The drawing under review shows one solid part. Ordinate dimensions are in mm from its lowest x, y, z. A direction names the side the tool comes from. Give positions to 0.01 mm unless a question says otherwise; leave off trailing zeros. Write each loop counter-clockwise with the first axis right and the second up, starting at its lowest first coordinate (ties: lowest second). Pieces come first, ordered by that corner, then holes. Notation, with made-up numbers: M 64.5,46.25 L 114.5,46.25 A23 ccw 114.5,60.25 Z; hole C -40,58 d2. An arc over 180 degrees is marked long. One line per item, written item: value. Start each with the question number.
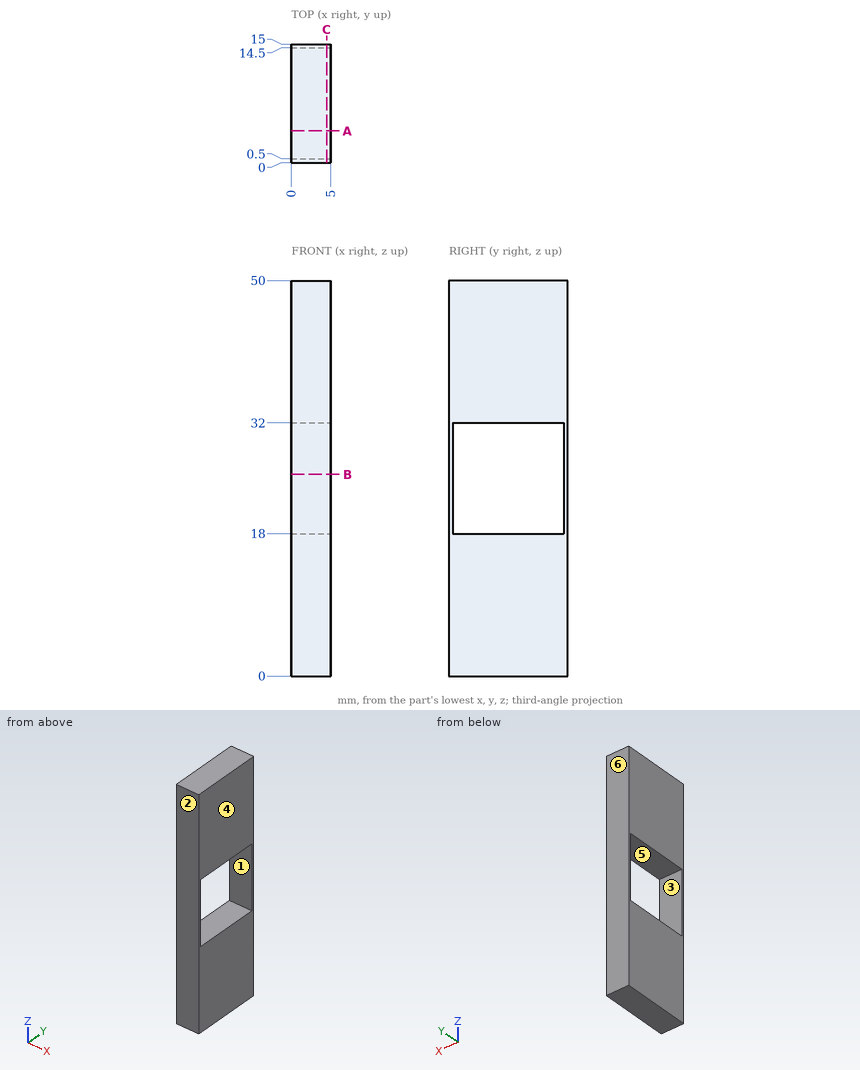
Q1. Take a section at B-B, the plane z = 25.5. Give the boundary of the cut face in (x, y).
Q2. For P1, Ø2, axis at y = 12, z = 39.5, coming from the -X side; P2, Ø1.5, axis at y = 5.5, z = 19, coming from the +X side, all flat-tipped, find the tip position at first contact; note any pin that passes through.
Q3. Take a section at C-C, the plane x = 4.45. Give the boundary of the cut face in (y, z), then the cut area to 3 significant figures.
Q4. Wall thickness on line 1 (Z direction, x = 4.35, y = 8.25); line 2 (Y direction, x = 4.1, z = 27): over which ranges is each line inside the solid? List them lowest first. Write a range as from..to.
Q5. The part is to be moulded in two halves that separate along Y. For the marked faces 1, 2, 3 and 4, say which applies: pulls with the +Y half, pulls with the -Y half, needs draft (parallel to the pull), parting line crosses it, or undercut.
Q6. Machinability: for the marked faces 5 and 6, which of the approach directions +Z, -Z, +X, -X, +Y, -Y give a long, thin tool a straight path to every point of the face, cutting with its end or side? Answer none if there is none.
Q7. Take a section at A-A, the plane y = 4. Give the boundary of the cut face in (x, z), then the cut area to 3 significant figures.
Results list:
1. outline: M 0,0 L 5,0 L 5,0.5 L 0,0.5 Z; M 0,14.5 L 5,14.5 L 5,15 L 0,15 Z
2. P1: stops at x = 0
2. P2: passes through
3. outline: M 0,0 L 15,0 L 15,50 L 0,50 Z; hole M 0.5,18 L 14.5,18 L 14.5,32 L 0.5,32 Z
3. area: 554 mm^2
4. line 1: z = 0..18, 32..50
4. line 2: y = 0..0.5, 14.5..15
5. face 1: undercut
5. face 2: pulls with the -Y half
5. face 3: undercut
5. face 4: needs draft
6. face 5: +X, -X
6. face 6: +Z, -Z, +X, -X, +Y
7. outline: M 0,0 L 5,0 L 5,18 L 0,18 Z; M 0,32 L 5,32 L 5,50 L 0,50 Z
7. area: 180 mm^2
